Here's the drawing with two shaded views (mm, measured from the low corner). I have some questions. A direction names the side the tool comes from. Coordinates: 2 decimals unless noted, no trailing zeros. Write each loop counter-clockwise with the first axis right and the second up, starting at its lowest first coordinate (ties: lowest second). Pieces come first, ordered by that corner, then holes. Notation, with made-up numbers: M 17.5,-0.5 L 56.5,-0.5 A11 ccw 56.5,12.5 Z; hole C 64,-29 d8. An arc over 180 degrees is marked long. Answer as CSV lines item,"result". Start each with the question number.
Item 1: I'm going to push flat-ended pins straight in: P1, Ø1.5, axis at y = 129.5, z = 18.5, coming from the +X side; P2, Ø12, axis at x = 178.5, y = 127.5, coming from the -Z side; P3, Ø16.5, axis at y = 131, z = 14, coming from the -X side. Where does each tip first touch, or does it pass through?
Item 2: Suppose I cut it at A-A, the plane x = 150. Write out the boundary of the cut face in (y, z), and give its area (4 significant figures).
Item 3: On a 3-axis mill with a long thin cutter (end or side, diameter ignored), from which of +Z, -Z, +X, -X, +Y, -Y can I reach the whole of each face in a straight line? I mean the marked faces 1, 2 and 3. Say none if no direction works.
Item 4: Suppose I cut it at C-C, the plane y = 125.5. Write out the boundary of the cut face in (x, z).
Item 5: Suppose I cut it at B-B, the plane y = 146. Write out the boundary of the cut face in (x, z).
Item 6: If I drill on line 1 along Z through (x, y) = (152, 132.5); line 2 along X through (y, z) = (150, 10); line 3 along X through (y, z) = (139.5, 15.5), over which ranges is the centre line in solid material (lowest first)? Write a range as [from, to].
Item 7: Suppose I cut it at D-D, the plane x = 86. Write out the boundary of the cut face in (y, z).
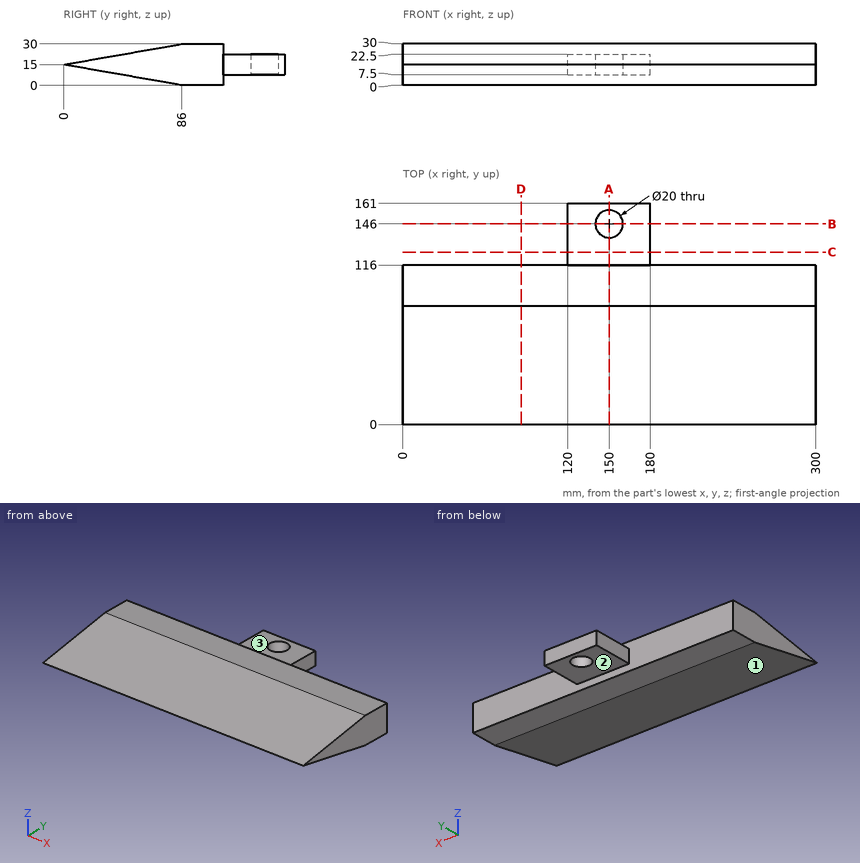
Ans:
1,P1,"stops at x = 180"
1,P2,"stops at z = 7.5"
1,P3,"stops at x = 120"
2,outline,"M 0,15 L 86,0 L 116,0 L 116,7.5 L 136,7.5 L 136,22.5 L 116,22.5 L 116,30 L 86,30 Z; M 156,7.5 L 161,7.5 L 161,22.5 L 156,22.5 Z"
2,area,"2,565 mm^2"
3,face 1,"-Z, +X, -X, -Y"
3,face 2,"-Z, +X, -X, +Y"
3,face 3,"+Z, +X, -X, +Y"
4,outline,"M 120,7.5 L 180,7.5 L 180,22.5 L 120,22.5 Z"
5,outline,"M 120,7.5 L 140,7.5 L 140,22.5 L 120,22.5 Z; M 160,7.5 L 180,7.5 L 180,22.5 L 160,22.5 Z"
6,line 1,"z = [7.5, 22.5]"
6,line 2,"x = [120, 140.83], [159.17, 180]"
6,line 3,"x = [120, 142.4], [157.6, 180]"
7,outline,"M 0,15 L 86,0 L 116,0 L 116,30 L 86,30 Z"
